Can you work these out from the model? Positions are in its coordinate system, mm. Face numbers are marked on the shaded views. A direction names the side the tool comes from. Round coordinates to 2 decimals unless told otherwise and drop trailing zeros. Order: outer loops, then holes, each group sorted by start corner. A loop starts at its lowest first (then second) coordinate and runs counter-clockwise, first axis right, second up.
Q1. If we section it at B-B (x = 10): Please give me the cut outline in (y, z), plus the area to 3 significant figures.
Q2. We'd pull the mould along X, two halves only. Please class the marked faces 4, 5, 6 and 7: pulls with the +X half, pulls with the -X half, needs draft (parallel to the pull), parting line crosses it, or undercut.
Q3. If I drill on line 1 (X direction, y = -13.5, z = -10); line 2 (Y direction, x = -34.5, z = -14); line 3 (X direction, y = -23.5, z = -25), over which ranges is the centre line in solid material (lowest first)?
Q4. Will these pins go through, and if not, where does the flat tip stop? P1, Ø0.8, axis at x = 7, y = -24.5, coming from the +Z side; P2, Ø10, axis at x = 19, y = -16, coming from the +Z side.
Q5. If we section it at A-A (z = -18): Count the separate pieces of the cut face and the enclosed holes in it, plus the area to 3 significant figures.
Q6. For the marked faces 1, 2 and 3, which set-ups out of +Z, -Z, +X, -X, +Y, -Y let a thin tool reach every point of the face, with its end or its side?
from build123d import *

# Parameters (mm, degrees)
F1_DEPTH      = 25.4
F2_T          = -2.54
F3_R          = 8.9609270722
F4_DEPTH      = 105.41
F5_SIZE       = 2.53999
F6_R          = 19.1294081244
F7_DEPTH      = 254
F7_DEPTH_BACK = 170.942


# Not quite as in the source:
# - a fillet or chamfer is up to 0.001 mm smaller than in the source, because OpenCascade refuses the exact size


with BuildPart() as f1:
    # F0 (on Front) → F1 (new body)
    with BuildSketch(Plane.XZ):
        Polygon((40.64, -40.64), (40.64, 0), (30.4068718106, 0), (15.24, -7.0667252876), (15.24, -33.4807746112), (-15.24, -33.4807746112), (-15.24, -7.0667252876), (-30.4068718106, 0), (-40.64, 0), (-40.64, -40.64), align=None)
        Polygon((-30.4068718106, 0), (-40.64, 40.64), (-40.64, 0), align=None)
        Polygon((40.64, 0), (40.64, 40.64), (30.4068718106, 0), align=None)
    extrude(amount=F1_DEPTH)

    # F2
    f2_openings = [f1.faces().sort_by_distance(p)[0] for p in [
        (35.523436, -12.7, 20.32),
        (22.823436, -12.7, -3.533363),
        (15.24, -12.7, -20.27375),
        (0, -12.7, -33.480775),
        (-35.523436, -12.7, 20.32),
        (-22.823436, -12.7, -3.533363),
        (-15.24, -12.7, -20.27375),
    ]]
    offset(amount=F2_T, openings=f2_openings)

    # F3 (on Front) → F4 (cut)
    with BuildSketch(Plane.XZ):
        with Locations((-29.5430510807, -23.22207205)):
            Circle(F3_R)
        with Locations((29.538249597, -23.22207205)):
            Circle(F3_R)
    extrude(amount=F4_DEPTH, mode=Mode.SUBTRACT)

    # F5 (size 2.54 in the source; OpenCascade refuses exactly that, so slightly less here)
    f5_edges = [f1.edges().sort_by_distance(p)[0] for p in [
        (-34.253436, -22.86, 15.276303),
        (-22.823436, -22.86, -3.533363),
        (-34.253436, -2.54, 15.276303),
        (-22.823436, -2.54, -3.533363),
        (22.823436, -2.54, -3.533363),
        (34.253436, -2.54, 15.276303),
        (34.253436, -22.86, 15.276303),
        (22.823436, -22.86, -3.533363),
    ]]
    chamfer(f5_edges, length=F5_SIZE)

    # F6 (on Right) → F7 (cut, two sides)
    with BuildSketch(Plane.YZ) as f7_sk:
        with Locations((-12.8998877481, 54.9755766988)):
            Circle(F6_R)
    extrude(amount=-F7_DEPTH, mode=Mode.SUBTRACT)
    extrude(f7_sk.sketch, amount=F7_DEPTH_BACK, mode=Mode.SUBTRACT)


solid = f1.part
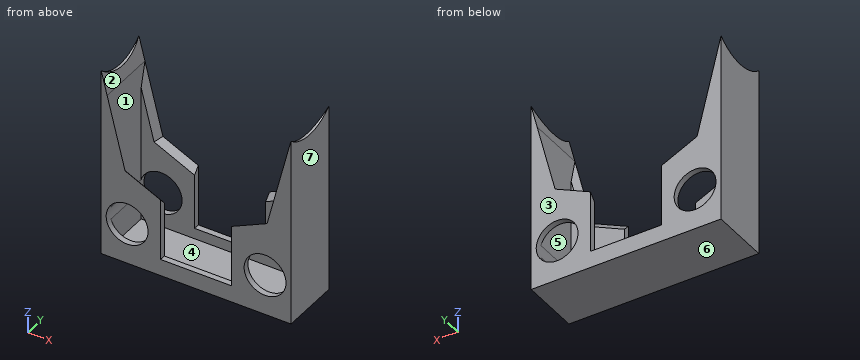
Solution:
1. outline: (-25.4, -40.64) - (0, -40.64) - (0, -33.48) - (-2.54, -33.48) - (-2.54, -38.1) - (-22.86, -38.1) - (-22.86, -33.48) - (-25.4, -33.48) - close
1. area: 88.0 mm2
2. face 4: undercut
2. face 5: undercut
2. face 6: needs draft
2. face 7: pulls with the +X half
3. line 1: x = -40.64 to -38.1, 38.1 to 40.64
3. line 2: y = -25.4 to -22.86, -2.54 to 0
3. line 3: x = -40.64 to -38.33, -20.76 to -15.24, 15.24 to 20.76, 38.32 to 40.64
4. P1: stops at z = -33.48
4. P2: stops at z = -38.1
5. separate pieces: 6
5. enclosed holes: 0
5. area: 213 mm2
6. face 1: +Z
6. face 2: +Z, +Y, -Y
6. face 3: +Z, -Z, +X, -X, +Y
